```python
from build123d import *
from build123d.topology import SkipClean

# Parameters (mm, degrees)
SKETCH1_W               = 50
SKETCH1_H               = 50
SKETCH1_R               = 16.3
SKETCH1_R_2             = 2.75
BOSS_EXTRUDE1_DEPTH     = 53.6
CUT_EXTRUDE1_DEPTH      = 66.015075175
CUT_EXTRUDE1_DEPTH_BACK = 66.015075175
SKETCH2_R               = 31.75
BOSS_EXTRUDE3_START     = 35
BOSS_EXTRUDE3_DEPTH     = 35
CUT_EXTRUDE6_DEPTH      = 76.433606209
CUT_EXTRUDE6_DEPTH_BACK = 10
SKETCH10_R              = 2.8
CUT_EXTRUDE8_DEPTH      = 35
BOSS_EXTRUDE4_START     = 3.5
SKETCH16_W              = 35
SKETCH16_H              = 28
SKETCH16_R              = 2.8
BOSS_EXTRUDE4_DEPTH     = 3.5


with BuildPart() as part:
    # Sketch1 → Boss-Extrude1 (new body)
    with BuildSketch(Plane.XY):
        with Locations((0, -2)):
            Rectangle(SKETCH1_W, SKETCH1_H)
        with Locations((0, -2)):
            Circle(SKETCH1_R, mode=Mode.SUBTRACT)
        with Locations((-20, 18)):
            Circle(SKETCH1_R_2, mode=Mode.SUBTRACT)
        with Locations((20, 18)):
            Circle(SKETCH1_R_2, mode=Mode.SUBTRACT)
        with Locations((20, -22)):
            Circle(SKETCH1_R_2, mode=Mode.SUBTRACT)
        with Locations((-20, -22)):
            Circle(SKETCH1_R_2, mode=Mode.SUBTRACT)
    extrude(amount=BOSS_EXTRUDE1_DEPTH)

    # Sketch2 → Cut-Extrude1 (cut, two sides: drawn at the far end of the back side and taken through both)
    with BuildSketch(Plane(origin=(0, 0, 0), x_dir=(0, 0, -1), z_dir=(1, 0, 0)).offset(-CUT_EXTRUDE1_DEPTH_BACK)):
        Circle(SKETCH2_R)
    extrude(amount=CUT_EXTRUDE1_DEPTH + CUT_EXTRUDE1_DEPTH_BACK, mode=Mode.SUBTRACT)

    # Sketch4 → Boss-Extrude3 (add)
    with SkipClean():  # the faces are left unmerged after this step: merging them gives an invalid solid
        with BuildSketch(Plane(origin=(25, 0, 0), x_dir=(0, 0, -1), z_dir=(1, 0, 0)).offset(BOSS_EXTRUDE3_START)):
            with BuildLine():
                Line((-53.6, 11), (-53.6, -17))
                Line((-53.6, -17), (-26.815340759, -17))
                ThreePointArc((-26.815340759, -17), (-31.573087709, -3.347033393), (-29.783594477, 11))
                Line((-29.783594477, 11), (-53.6, 11))
            make_face()
        extrude(amount=-BOSS_EXTRUDE3_DEPTH)

    # Sketch10 → Cut-Extrude6 (cut, two sides: drawn at the far end of the back side and taken through both)
    with SkipClean():  # the faces are left unmerged after this step: merging them gives an invalid solid
        with BuildSketch(Plane.XY.offset(53.6).offset(-CUT_EXTRUDE6_DEPTH_BACK)):
            with Locations(Location((50, 4.5, 0), (0, 0, 180))):
                Circle(SKETCH10_R)
            with Locations(Location((50, -8.5, 0), (0, 0, 180))):
                Circle(SKETCH10_R)
        extrude(amount=CUT_EXTRUDE6_DEPTH + CUT_EXTRUDE6_DEPTH_BACK, mode=Mode.SUBTRACT)

    # Sketch13 → Cut-Extrude8 (cut)
    with BuildSketch(Plane(origin=(60, 0, 0), x_dir=(0, 0, -1), z_dir=(1, 0, 0))):
        with BuildLine():
            Line((-29.783594477, 11), (-40, 11))
            Line((-40, 11), (-40, -17))
            Line((-40, -17), (-26.815340759, -17))
            ThreePointArc((-26.815340759, -17), (-31.573087709, -3.347033393), (-29.783594477, 11))
        make_face()
    extrude(amount=-CUT_EXTRUDE8_DEPTH, mode=Mode.SUBTRACT)

    # Sketch16 → Boss-Extrude4 (add)
    with BuildSketch(Plane.XY.offset(53.6).offset(BOSS_EXTRUDE4_START)):
        with Locations((42.5, -3)):
            Rectangle(SKETCH16_W, SKETCH16_H)
        with Locations(Location((50, 4.5, 0), (0, 0, 180))):
            Circle(SKETCH16_R, mode=Mode.SUBTRACT)
        with Locations(Location((50, -8.5, 0), (0, 0, 180))):
            Circle(SKETCH16_R, mode=Mode.SUBTRACT)
    extrude(amount=-BOSS_EXTRUDE4_DEPTH)


solid = part.part
```
Can you work these out from the model? Positions are in its coordinate system, mm. A direction names the side the tool comes from. Coordinates: 2 decimals unless noted, no trailing zeros. Loops run counter-clockwise (first coordinate to the right, second up) from the corner with the lowest first, then second, coordinate; pieces in that order, holes last. Notation, with made-up numbers: M 64,27 L 93,27 A34 cw 93,57 Z; hole C -8.75,-17 d6. An arc over 180 degrees is marked long. Put each result on its own line as item: value. Start each with the question number.
(1) Will these pins go through, and if not, where does the flat tip stop? pin 1 Ø12 at (x, y) = (49.5, -1.5) entering from -Z; pin 2 Ø3 at (x, z) = (46, 41) entering from +Y; pin 3 Ø6.5 at (x, y) = (-20, -22) entering from -Z.
(2) Imagine slicing it at C-C on x = 50. List the corners of the cut face in (y, z) for me.
(3) I need wall thicknesses on probe 1 along X at (y, z) = (-22, 47.5); probe 2 along Y at (x, z) = (20, 35); probe 3 along Y at (x, z) = (50, 54). Which ranges of each line are inside material? Lowest first, please.
(4) Which directions (+Z, -Z, +X, -X, +Y, -Y) give clear straight access to the entire face, cutting with the end or side of a thin tool? Please do faces 1 (the face through (43, -3, 40)), 2 (the face through (42, -17, 49)), 3 (the face through (-17, -2, 53.6)).
(5) Imagine slicing it at A-A on z = 33. List the corners of the cut face in (x, y) for me.
(6) Imagine slicing it at D-D on x = -9.5. List the corners of the cut face in (y, z) for me, and give its area (3 significant figures).
(7) We'd pull the mould along Y, two halves only. Please class faces 4 (the face through (0, -27, 35)), 5 (the face through (42, -3, 57.1)), 6 (the face through (-3.534, -17.912, 42.651)), 7 (the face through (50, 4, 43.6)): +Y half, -Y half, draft (parallel to the pull), parting line (faces both ways), or undercut.
(8) Imagine slicing it at B-B on y = 10. List the corners of the cut face in (x, z) for me, and give its area (3 significant figures).
Worked answers:
1. pin 1: stops at z = 40
1. pin 2: stops at y = 11
1. pin 3: stops at z = 19.25
2. outline: M -17,40 L 11,40 L 11,57.1 L 7.3,57.1 L 7.3,43.6 L 1.7,43.6 L 1.7,57.1 L -5.7,57.1 L -5.7,43.6 L -11.3,43.6 L -11.3,57.1 L -17,57.1 Z
3. probe 1: x = -25 to -22.75, -17.25 to 17.25, 22.75 to 25
3. probe 2: y = -27 to -24.75, -19.25 to 15.25, 20.75 to 23
3. probe 3: y = -17 to -11.3, -5.7 to 1.7, 7.3 to 11
4. face 1: -Z, +X, +Y, -Y
4. face 2: +Z, -Z, +X, -Y
4. face 3: +Z, -X, +Y, -Y
5. outline: M -25,-27 L 25,-27 L 25,23 L -25,23 Z; hole C -20,-22 d5.5; hole C -20,18 d5.5; hole C 0,-2 d32.6; hole C 20,-22 d5.5; hole C 20,18 d5.5
6. outline: M -27,16.71 A31.75 cw -15.25,27.85 L -15.25,53.6 L -27,53.6 Z; M 11.25,29.69 A31.75 cw 23,21.89 L 23,53.6 L 11.25,53.6 Z
6. area: 676 mm2
7. face 4: -Y half
7. face 5: draft
7. face 6: undercut
7. face 7: undercut
8. outline: M -25,30.13 L -11.03,30.13 L -11.03,53.6 L -25,53.6 Z; M 11.03,30.13 L 25,30.13 L 25,40 L 60,40 L 60,57.1 L 25,57.1 L 25,53.6 L 11.03,53.6 Z
8. area: 1,250 mm2
